```python
from build123d import *

# Parameters (mm, degrees)
SKETCH3_R                = 1.25
SKETCH3_R_2              = 1.5
BOSS_EXTRUDE9_DEPTH      = 5
SKETCH4_R                = 7.5
BOSS_EXTRUDE10_DEPTH     = 4
SKETCH5_R                = 10
BOSS_EXTRUDE11_DEPTH     = 5
SKETCH6_R                = 1.5
CUT_EXTRUDE1_DEPTH       = 33.778193971
SKETCH7_W                = 12
SKETCH7_H                = 4
BOSS_EXTRUDE12_DEPTH     = 17
SKETCH8_W                = 3
SKETCH8_H                = 8
BOSS_EXTRUDE13_DEPTH     = 4
F_3_0_3_DIAMETER_HOLE1_D = 3


with BuildPart() as part:
    # Sketch3 → Boss-Extrude9 (new body)
    with BuildSketch(Plane(origin=(0, 0, 0), x_dir=(1, 0, 0), z_dir=(0, 1, 0))):
        with BuildLine():
            Line((24.1, 3.8), (8.85, 3.8))
            ThreePointArc((8.85, 3.8), (7.033595607, 4.14837388), (5.468099348, 5.133214346))
            ThreePointArc((5.468099348, 5.133214346), (-7.5, 0), (5.468099348, -5.133214346))
            ThreePointArc((5.468099348, -5.133214346), (7.033595607, -4.14837388), (8.85, -3.8))
            Line((8.85, -3.8), (24.1, -3.8))
            ThreePointArc((24.1, -3.8), (27.9, 0), (24.1, 3.8))
        make_face()
        with Locations(Location((8.85, 0, 0), (0, 0, 270))):
            Circle(SKETCH3_R, mode=Mode.SUBTRACT)
        with Locations(Location((20.1, 0, 0), (0, 0, 270))):
            Circle(SKETCH3_R_2, mode=Mode.SUBTRACT)
        with Locations(Location((24.1, 0, 0), (0, 0, 270))):
            Circle(SKETCH3_R_2, mode=Mode.SUBTRACT)
    extrude(amount=BOSS_EXTRUDE9_DEPTH)

    # Sketch4 → Boss-Extrude10 (add)
    with BuildSketch(Plane(origin=(0, 5, 0), x_dir=(1, 0, 0), z_dir=(0, 1, 0))):
        with Locations(Location((0, 0, 0), (0, 0, 43.19068472))):
            Circle(SKETCH4_R)
    extrude(amount=BOSS_EXTRUDE10_DEPTH)

    # Sketch5 → Boss-Extrude11 (add)
    with BuildSketch(Plane(origin=(0, 9, 0), x_dir=(1, 0, 0), z_dir=(0, 1, 0))):
        with Locations(Location((0, 0, 0), (0, 0, 270))):
            Circle(SKETCH5_R)
    extrude(amount=BOSS_EXTRUDE11_DEPTH)

    # Sketch6 → Cut-Extrude1 (cut, through all)
    with BuildSketch(Plane(origin=(0, 14, 0), x_dir=(1, 0, 0), z_dir=(0, 1, 0))):
        with Locations(Location((0, 0, 0), (0, 0, 270))):
            Circle(SKETCH6_R)
    extrude(amount=-CUT_EXTRUDE1_DEPTH, mode=Mode.SUBTRACT)

    # Sketch7 → Boss-Extrude12 (add)
    with BuildSketch(Plane(origin=(0, 14, 0), x_dir=(1, 0, 0), z_dir=(0, 1, 0))):
        with Locations((0, -6)):
            Rectangle(SKETCH7_W, SKETCH7_H)
        with Locations((0, 6)):
            Rectangle(SKETCH7_W, SKETCH7_H)
    extrude(amount=BOSS_EXTRUDE12_DEPTH)

    # Sketch8 → Boss-Extrude13 (add)
    with BuildSketch(Plane(origin=(0, 14, 0), x_dir=(1, 0, 0), z_dir=(0, 1, 0))):
        with Locations((4.5, 0)):
            Rectangle(SKETCH8_W, SKETCH8_H)
        with Locations((-4.5, 0)):
            Rectangle(SKETCH8_W, SKETCH8_H)
    extrude(amount=BOSS_EXTRUDE13_DEPTH)

    # 3.0 _3_ Diameter Hole1 (through all)
    with Locations(Plane.XY.offset(8)):
        with Locations((0, 28), (0, 22)):
            Hole(F_3_0_3_DIAMETER_HOLE1_D / 2)


solid = part.part
```
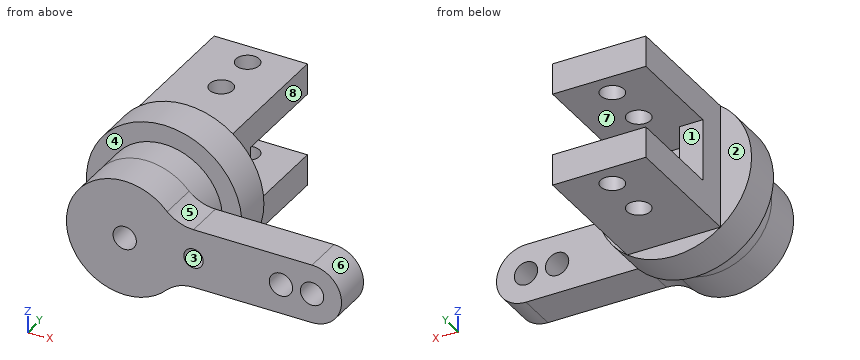
Build history of the part. All positions in model axes, mm. Face numbers are marked on the shaded views. A direction names the side the tool comes from. Coordinates: 2 decimals unless noted, no trailing zeros. Order: outer loops, then holes, each group sorted by start corner. A loop starts at its lowest first (then second) coordinate and runs counter-clockwise, first axis right, second up. Notation, with made-up numbers: (79, 20.25) -> (88, 20.25) arc R37 ccw to (88, 58.25) -> close; hole circle Ø5 at (88, 83.5). An arc over 180 degrees is marked (long way). Answer in a Markdown table with one row per item. Add a question column.
Q1. Wall check: line 1 along Y through (x, z) = (0, -5.05); line 2 along Z through (x, y) = (2.5, 17.5); line 3 along Y through (x, z) = (-2, 3.25). Give the ranges that are in metal, low to high. Write a range as [from, to].
Q2. Which spindle directions (+Z, -Z, +X, -X, +Y, -Y) get a long thin tool onto all of the face, cutting with end or side? Do the marked faces 1, 2, 3, 4 and 5. Say none if no direction does.
Q3. Band-saw the part on B-B, the plane y = 22. List the corners of the cut face in (x, z), then the cut area to 3 significant figures.
Q4. Band-saw the part on D-D, the plane z = 5.75. List the corners of the cut face in (x, y), then the cut area to 3 significant figures.
Q5. Band-saw the part on A-A, the plane z = 0. Give the number of separate pieces and of enclosed holes in the cut face, then the cut area to 4 significant figures.
Q6. Drop flat-ended pins along their axis: pin 1 (5 mm diameter, centred on x = 0, y = 28, fed in from -Z); pin 2 (8 mm diameter, centred on y = 23, z = 1, fed in from -X); pin 3 (1 mm diameter, centred on y = 12, z = -4, fed in from -X); pin 4 (1.8 mm diameter, centred on x = 0, y = 22, fed in from -Z). Give the stop position or say it passes through.
Q7. Mould opens along Z. For the marked faces 6, 7 and 8 say: +Z half, -Z half, draft (parallel to the pull), parting line (faces both ways), or undercut.
Answers follow:
| question | item | result |
|---|---|---|
| 1 | line 1 | [0, 20.5], [23.5, 26.5], [29.5, 31] |
| 1 | line 2 | [-8, -4], [4, 8] |
| 1 | line 3 | [0, 14] |
| 2 | face 1 | +X, -X, +Y |
| 2 | face 2 | +Z, -Z, -X, +Y |
| 2 | face 3 | -Y |
| 2 | face 4 | none |
| 2 | face 5 | +Z, +X, -Y |
| 3 | outline | (-6, -8) -> (-1.5, -8) -> (-1.5, -4) -> (-6, -4) -> close; (-6, 4) -> (-1.5, 4) -> (-1.5, 8) -> (-6, 8) -> close; (1.5, -8) -> (6, -8) -> (6, -4) -> (1.5, -4) -> close; (1.5, 4) -> (6, 4) -> (6, 8) -> (1.5, 8) -> close |
| 3 | area | 72.0 mm^2 |
| 4 | outline | (-8.18, 9) -> (-4.82, 9) -> (-4.82, 0) -> (4.82, 0) -> (4.82, 9) -> (8.18, 9) -> (8.18, 14) -> (6, 14) -> (6, 31) -> (-6, 31) -> (-6, 14) -> (-8.18, 14) -> close; hole circle Ø3 at (0, 22); hole circle Ø3 at (0, 28) |
| 4 | area | 358 mm^2 |
| 5 | separate pieces | 5 |
| 5 | enclosed holes | 0 |
| 5 | area | 276.5 mm^2 |
| 6 | pin 1 | z = -8 |
| 6 | pin 2 | x = -6 |
| 6 | pin 3 | x = -9.37 |
| 6 | pin 4 | through |
| 7 | face 6 | parting line |
| 7 | face 7 | undercut |
| 7 | face 8 | draft |
